```python
from build123d import *

# Parameters (mm, degrees)
SKETCH1_W                   = 55
SKETCH1_H                   = 27
SKETCH1_W_2                 = 38.1
SKETCH1_H_2                 = 5
BOTTOM_BASE_DEPTH           = 3
SENSOR_MOUNTING_HOLES_DEPTH = 3
SKETCH4_W                   = 55
SKETCH4_H                   = 27
SKETCH4_W_2                 = 53
SKETCH4_H_2                 = 25
SKETCH4_W_3                 = 7
SKETCH4_H_3                 = 7
OUTER_RIM_DEPTH             = 3
M4_BOLT_HOLES_D             = 5
BACKWARDS_SENSOR_DEPTH      = 3


with BuildPart() as part:
    # Sketch1 → Bottom Base (new body)
    with BuildSketch(Plane(origin=(0, 0, 0), x_dir=(1, 0, 0), z_dir=(0, 1, 0))):
        Rectangle(SKETCH1_W, SKETCH1_H)
        with Locations((0, -5.25)):
            Rectangle(SKETCH1_W_2, SKETCH1_H_2, mode=Mode.SUBTRACT)
        with Locations((0, 3.5)):
            Rectangle(SKETCH1_W_2, SKETCH1_H_2, mode=Mode.SUBTRACT)
    extrude(amount=BOTTOM_BASE_DEPTH)

    # Sketch3 → Sensor Mounting Holes (cut)
    with BuildSketch(Plane(origin=(0, 3, 0), x_dir=(1, 0, 0), z_dir=(0, 1, 0))):
        with BuildLine():
            Line((-14.5, 10.1), (14.500000132, 10.1))
            ThreePointArc((14.500000132, 10.1), (15.750000132, 8.85), (14.500000132, 7.6))
            Line((14.500000132, 7.6), (-14.5, 7.6))
            ThreePointArc((-14.5, 7.6), (-15.75, 8.85), (-14.5, 10.1))
        make_face()
    extrude(amount=-SENSOR_MOUNTING_HOLES_DEPTH, mode=Mode.SUBTRACT)

    # Sketch4 → Outer Rim (add)
    with BuildSketch(Plane(origin=(0, 3, 0), x_dir=(1, 0, 0), z_dir=(0, 1, 0))):
        Rectangle(SKETCH4_W, SKETCH4_H)
        Rectangle(SKETCH4_W_2, SKETCH4_H_2, mode=Mode.SUBTRACT)
        with Locations((23, 9)):
            Rectangle(SKETCH4_W_3, SKETCH4_H_3)
        with Locations((23, -9)):
            Rectangle(SKETCH4_W_3, SKETCH4_H_3)
        with Locations((-23, -9)):
            Rectangle(SKETCH4_W_3, SKETCH4_H_3)
        with Locations((-23, 9)):
            Rectangle(SKETCH4_W_3, SKETCH4_H_3)
    extrude(amount=OUTER_RIM_DEPTH)

    # M4 bolt holes (through all)
    with Locations(Plane(origin=(0, 6, 0), x_dir=(1, 0, 0), z_dir=(0, 1, 0))):
        with Locations((-23.5, 9.5), (-23.5, -9.5), (23.5, 9.5), (23.5, -9.5)):
            Hole(M4_BOLT_HOLES_D / 2)

    # Sketch11 → backwards sensor (cut)
    with BuildSketch(Plane(origin=(0, 3, 0), x_dir=(1, 0, 0), z_dir=(0, 1, 0))):
        with BuildLine():
            Line((-7.5, -9.25), (7.5, -9.25))
            ThreePointArc((7.5, -9.25), (8.75, -10.5), (7.5, -11.75))
            Line((7.5, -11.75), (-7.5, -11.75))
            ThreePointArc((-7.5, -11.75), (-8.75, -10.5), (-7.5, -9.25))
        make_face()
    extrude(amount=-BACKWARDS_SENSOR_DEPTH, mode=Mode.SUBTRACT)


solid = part.part
```
Model file for the job. Use its own axes, mm. A direction names the side the tool comes from. Give positions to 0.01 mm unless a question says otherwise; leave off trailing zeros. Loops run counter-clockwise (first coordinate to the right, second up) from the corner with the lowest first, then second, coordinate; pieces in that order, holes last. Notation, with made-up numbers: (21.5, 1) -> (35.5, 1) arc R22 ccw to (35.5, 30) -> close; hole circle Ø6 at (-14.5, 60.5). An arc over 180 degrees is marked (long way). Write each question's results on one line, items separated by ' | '.
(1) Flat gauge pins, fed straight in: pin 1 Ø6 at (x, z) = (-1.5, -7.5) entering from +Y; pin 2 Ø8 at (x, z) = (23.5, 9.5) entering from -Y. Where does each tip first touch, or does it go through?
Geometry results:
pin 1: stops at y = 3 | pin 2: stops at y = 0
(2) Cut at D-D on z = 10.5. List the corners of the cut face in (x, y), and give its area (3 significant figures).
Geometry results:
outline: (-27.5, 0) -> (-25.79, 0) -> (-25.79, 6) -> (-27.5, 6) -> close; (-21.21, 0) -> (-8.75, 0) -> (-8.75, 3) -> (-19.5, 3) -> (-19.5, 6) -> (-21.21, 6) -> close; (8.75, 0) -> (21.21, 0) -> (21.21, 6) -> (19.5, 6) -> (19.5, 3) -> (8.75, 3) -> close; (25.79, 0) -> (27.5, 0) -> (27.5, 6) -> (25.79, 6) -> close | area: 106 mm²
(3) Cut at B-B on y = 1.85. Give the number of separate pieces and of enclosed holes in the cut face, and give its area (3 significant figures).
Geometry results:
separate pieces: 1 | enclosed holes: 8 | area: 906 mm²
(4) Probe line 1 along Z through (x, y) = (-23.5, 1.95); line 2 along Z through (x, y) = (-14.5, 1.7); line 3 along Z through (x, y) = (23.5, 3.55). List the from-to ranges inside material, lowest first.
Geometry results:
line 1: z = -13.5 to -12, -7 to 7, 12 to 13.5 | line 2: z = -13.5 to -10.1, -7.6 to -6, -1 to 2.75, 7.75 to 13.5 | line 3: z = -13.5 to -12, -7 to -5.5, 5.5 to 7, 12 to 13.5
(5) Tool access for faces 1 (the flat face through (19.5, 4, 9)), 2 (the flat face through (0, 1, 7.75)), 3 (the flat face through (0, 0, 0)): list every direction of +Z, -Z, +X, -X, +Y, -Y with a clear straight run to the whole face (end or side of a thin tool).
Geometry results:
face 1: +Y | face 2: +Y, -Y | face 3: +Z, -Z, +X, -X, -Y
(6) Pull direction Z, two halves, no side cores. Call faces 4 (the flat face through (0, 6, 13)), 5 (the flat face through (23, 4, -5.5)), 6 (the flat face through (19.05, 1, 5)): released by +Z, released by -Z, zero draft, split by the parting line, or undercut.
Geometry results:
face 4: zero draft | face 5: undercut | face 6: undercut
(7) Cut at C-C on x = -11. List the corners of the cut face in (y, z), and give its area (3 significant figures).
Geometry results:
outline: (0, -13.5) -> (6, -13.5) -> (6, -12.5) -> (3, -12.5) -> (3, -10.1) -> (0, -10.1) -> close; (0, -7.6) -> (3, -7.6) -> (3, -6) -> (0, -6) -> close; (0, -1) -> (3, -1) -> (3, 2.75) -> (0, 2.75) -> close; (0, 7.75) -> (3, 7.75) -> (3, 12.5) -> (6, 12.5) -> (6, 13.5) -> (0, 13.5) -> close | area: 49.5 mm²
(8) Cut at A-A on x = -23.5. List the corners of the cut face in (y, z).
Geometry results:
outline: (0, -13.5) -> (6, -13.5) -> (6, -12) -> (0, -12) -> close; (0, -7) -> (6, -7) -> (6, -5.5) -> (3, -5.5) -> (3, 5.5) -> (6, 5.5) -> (6, 7) -> (0, 7) -> close; (0, 12) -> (6, 12) -> (6, 13.5) -> (0, 13.5) -> close
